Can you work these out from the drawing? Everything is in mm from the part's minimum corner. A direction names the side the tool comes from. Round coordinates to 2 decimals unless told otherwise and drop trailing zeros. Order: outer loops, then holes, each group sorted by start corner. A loop starts at its lowest first (then second) coordinate and runs counter-clockwise, first axis right, second up. Notation, with made-up numbers: M 80.25,27 L 85.25,27 A32 ccw 85.25,57 Z; hole C 13.25,5 d8. An arc over 180 degrees is marked long. Answer as a JSON object with one key per item and string values. Group by question number.
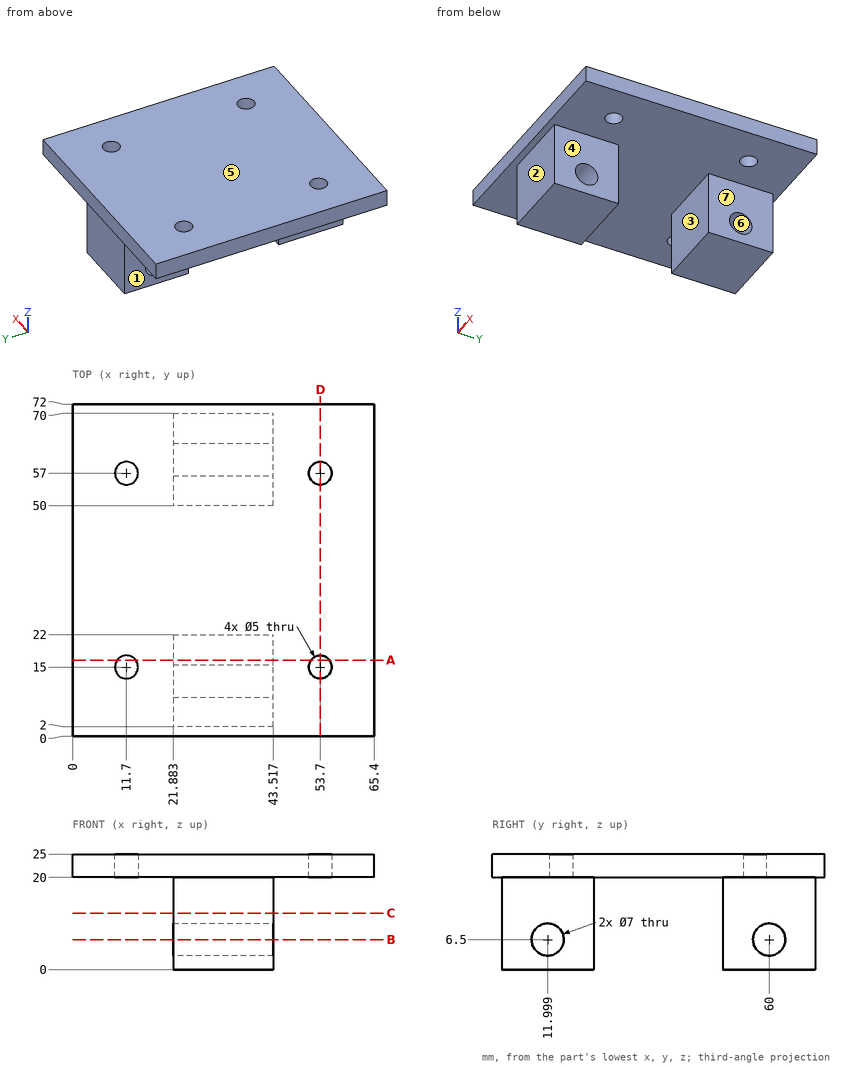
Item 1: Suppose I cut it at C-C, the plane z = 12.25. Write out the boundary of the cut face in (x, y).
Item 2: On a 3-axis mill with a long thin cutter (end or side, diameter ignored), from which of +Z, -Z, +X, -X, +Y, -Y can I reach the whole of each face in a straight line? I mean the marked faces 1, 2, 3 and 4. Say none if no direction works.
Item 3: Suppose I cut it at A-A, the plane y = 16.5. Write out the boundary of the cut face in (x, z), and give its area (3 significant figures).
Item 4: If we mould it in two halves opening along Z, with no side actions, what happens to the marked faces 5, 6 and 7? For each: +Z half, -Z half, draft (parallel to the pull), parting line (faces both ways), or undercut.
Item 5: I need wall thicknesses on line 1 (Y direction, x = 32.5, z = 6.5); line 2 (Y direction, x = 53.7, z = 23.7); line 3 (X direction, y = 56.5, z = 23.5). Which ranges of each line are inside material? Lowest first, please.
Item 6: Suppose I cut it at B-B, the plane z = 6.5. Write out the boundary of the cut face in (x, y).
Item 7: Suppose I cut it at D-D, the plane x = 53.7. Write out the boundary of the cut face in (y, z), and give its area (3 significant figures).
Item 8: I'm going to push flat-ended pins straight in: pin 1 Ø6 at (x, z) = (29.5, 15) entering from +Y; pin 2 Ø10 at (x, z) = (29, 14.5) entering from -Y; pin 3 Ø12 at (x, y) = (43.5, 13.5) entering from -Z; pin 4 Ø6 at (y, z) = (62, 8) entering from +X. Where does each tip first touch, or does it pass through?
Computed:
{
 "1": {"outline": "M 21.88,2 L 43.52,2 L 43.52,22 L 21.88,22 Z; M 21.88,50 L 43.52,50 L 43.52,70 L 21.88,70 Z"},
 "2": {"face 1": "-Z, -X, +Y, -Y", "face 2": "-Z, +X, -X, -Y", "face 3": "-Z, +X, -X", "face 4": "-Z, +X, +Y, -Y"},
 "3": {"outline": "M 0,20 L 9.7,20 L 9.7,25 L 0,25 Z; M 13.7,20 L 21.88,20 L 21.88,0 L 43.52,0 L 43.52,20 L 51.7,20 L 51.7,25 L 13.7,25 Z; M 55.7,20 L 65.4,20 L 65.4,25 L 55.7,25 Z", "area": "720 mm^2"},
 "4": {"face 5": "+Z half", "face 6": "undercut", "face 7": "draft"},
 "5": {"line 1": "y = 2 to 8.5, 15.5 to 22, 50 to 56.5, 63.5 to 70", "line 2": "y = 0 to 12.5, 17.5 to 54.5, 59.5 to 72", "line 3": "x = 0 to 9.25, 14.15 to 51.25, 56.15 to 65.4"},
 "6": {"outline": "M 21.88,2 L 43.52,2 L 43.52,8.5 L 21.88,8.5 Z; M 21.88,15.5 L 43.52,15.5 L 43.52,22 L 21.88,22 Z; M 21.88,50 L 43.52,50 L 43.52,56.5 L 21.88,56.5 Z; M 21.88,63.5 L 43.52,63.5 L 43.52,70 L 21.88,70 Z"},
 "7": {"outline": "M 0,20 L 12.5,20 L 12.5,25 L 0,25 Z; M 17.5,20 L 54.5,20 L 54.5,25 L 17.5,25 Z; M 59.5,20 L 72,20 L 72,25 L 59.5,25 Z", "area": "310 mm^2"},
 "8": {"pin 1": "stops at y = 70", "pin 2": "stops at y = 2", "pin 3": "stops at z = 0", "pin 4": "stops at x = 43.52"}
}
